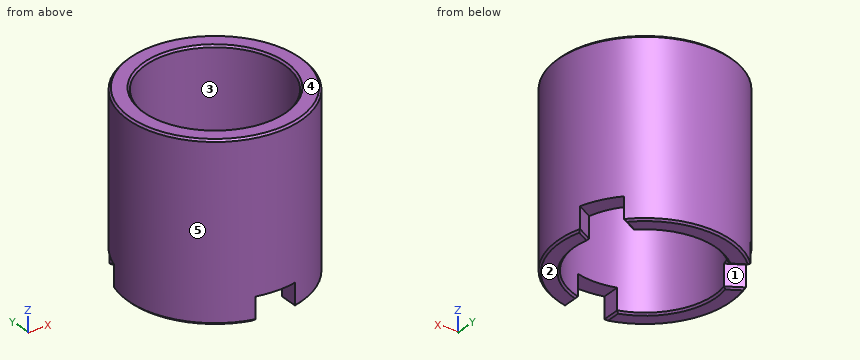
from build123d import *

# Parameters (mm, degrees)
F0_R     = 23.8125
F0_R_2   = 19.05
F1_DEPTH = 47.625
F2_W     = 10.795
F2_H     = 5.5431405764
F3_DEPTH = 6.35
F4_SIZE  = 0.508


with BuildPart() as f1:
    # F0 (on Top) → F1 (new body)
    with BuildSketch(Plane.XY):
        Circle(F0_R)
        Circle(F0_R_2, mode=Mode.SUBTRACT)
    extrude(amount=F1_DEPTH)

    # F2 (on face) → F3 (cut)
    with BuildSketch(Plane(origin=(0, 0, 0), x_dir=(1, 0, 0), z_dir=(0, 0, -1))):
        with Locations((0, 21.0409297118)):
            Rectangle(F2_W, F2_H)
        Polygon((-23.3209799276, -7.2318778831), (-17.9234799276, -16.5806221169), (-13.1229793717, -13.8090518287), (-18.5204793717, -4.4603075949), align=None)
        Polygon((17.9234799276, -16.5806221169), (23.3209799276, -7.2318778831), (18.5204793717, -4.4603075949), (13.1229793717, -13.8090518287), align=None)
    extrude(amount=-F3_DEPTH, mode=Mode.SUBTRACT)

    # F4
    f4_edges = [f1.edges().sort_by_distance(p)[0] for p in [
        (-23.8125, 0, 47.625),
        (-19.05, 0, 47.625),
        (-16.497784, -9.525, 0),
        (-20.62223, -11.90625, 0),
        (18.648902, -14.807214, 0),
        (15.259831, -11.403511, 0),
        (0, 19.05, 0),
        (0, 23.8125, 0),
        (-20.652356, 5.691147, 0),
        (-5.3975, -20.731039, 0),
        (5.3975, -20.731039, 0),
        (20.652356, 5.691147, 0),
        (15.254856, 15.039891, 0),
        (-15.254856, 15.039891, 0),
    ]]
    chamfer(f4_edges, length=F4_SIZE)


solid = f1.part
Work out the finished part from the listing and answer in its coordinate system (mm). Face numbers are marked on the shaded views. A direction names the side the tool comes from. Give positions to 0.01 mm unless a question says otherwise; leave off trailing zeros. Answer in a Markdown table with one row per item. Add a question column.
Q1. Determine the mould class of the marked faces 3, 4 and 5 for opening direction Y: released by +Y, released by -Y, zero draft, split by the parting line, or undercut.
Q2. Consider line 1 along Y through (x, z) = (0, 10); line 2 along X through (y, z) = (-6, 28.5). Determine where each line is inside the solid, lowest interval first.
Q3. A tool of negligible diameter and unlimited length cuts with its end or side. For the marked faces 1 and 2, from which of +Z, -Z, +X, -X, +Y, -Y can it reach the whole face along a straight path? Write none if from no direction.
Q4. Each of these flat-tipped pins is pushed along its axis until it touches: P1, Ø1.5, axis at x = 10.5, z = 36.5, coming from the -Y side; P2, Ø4, axis at y = -20.5, z = 4.5, coming from the -X side; P3, Ø1.5, axis at y = -22, z = 4, coming from the +X side. Where does it stop, or does it pass through?
Q5. The part is cut by section C-C (z = 4). State how many separate pieces and enclosed holes the cut face has, and give its area (3 significant figures).
Solution:
| question | item | result |
|---|---|---|
| 1 | face 3 | undercut |
| 1 | face 4 | zero draft |
| 1 | face 5 | split by the parting line |
| 2 | line 1 | y = -23.81 to -19.05, 19.05 to 23.81 |
| 2 | line 2 | x = -23.04 to -18.08, 18.08 to 23.04 |
| 3 | face 1 | -Z, +Y |
| 3 | face 2 | -Z, +X, -X, +Y, -Y |
| 4 | P1 | stops at y = -21.72 |
| 4 | P2 | stops at x = -14.99 |
| 4 | P3 | stops at x = 10.75 |
| 5 | separate pieces | 3 |
| 5 | enclosed holes | 0 |
| 5 | area | 485 mm² |
